Verification items for the finished model (mm, model axes). A direction names the side the tool comes from. Give positions to 0.01 mm unless a question says otherwise; leave off trailing zeros. Loops run counter-clockwise (first coordinate to the right, second up) from the corner with the lowest first, then second, coordinate; pieces in that order, holes last. Notation, with made-up numbers: (74, 78.25) - (83, 78.25) arc R19 cw to (83, 95.25) - close; hole circle Ø9 at (-2.75, -27). An arc over 180 degrees is marked (long way). One line per item, written item: value. Start each with the question number.
1. Scan lines: L1, parallel to X at y = -0.1, z = 4; L2, parallel to Z at x = 14, y = -0.7; L3, parallel to Z at x = 13, y = 0. Record each from-to range of solid material in increasing order. Write a range as [from, to].
2. Sectioned sample at A-A (x = 14). Record the cut outline in (y, z), plus the area to 3 significant figures.
3. Sectioned sample at D-D (x = 7). Record the cut outline in (y, z).
4. Access from +Z, -Z, +X, -X, +Y, -Y to the whole of each face (thin tool, end or side, straight path). Record for faces 4 (the cylindrical face through (-2.44, 7.94, -0.54)), 5 (the flat face through (16.5, 0, 0)).
5. Sectioned sample at B-B (z = -5.5). Record the cut outline in (x, y), plus the area to 3 significant figures.
6. Mould release check, pull along Z, two halves, no side actions. Record for faces 1 (the flat face through (0, 12, 0)), 2 (the cylindrical face through (-12.648, 0.028, -5.474)), 3 (the flat face through (0, 0, 10)): pulls with the +Z half, pulls with the -Z half, needs draft (parallel to the pull), parting line crosses it, or undercut.
7. Sectioned sample at C-C (y = 5.25). Record the cut outline in (x, z), plus the area to 3 significant figures.
8. Gauge pin test, flat end, axial feed: pin 1 (10 mm diameter, centred on x = 7.5, z = -6, fed in from +Y). Record the tip position at first contact, or that the pin passes through.
from build123d import *

# Parameters (mm, degrees)
SKETCH1_W           = 33
SKETCH1_H           = 20
BOSS_EXTRUDE1_DEPTH = 2
SKETCH2_R           = 2
CUT_EXTRUDE1_DEPTH  = 20.704060495
SKETCH3_R           = 2.5
BOSS_EXTRUDE2_DEPTH = 10
FILLET1_SIZE        = 2


with BuildPart() as part:
    # Sketch1 → Boss-Extrude1 (new, symmetric)
    with BuildSketch(Plane(origin=(0, 0, 0), x_dir=(1, 0, 0), z_dir=(0, 1, 0))):
        Rectangle(SKETCH1_W, SKETCH1_H)
    extrude(amount=BOSS_EXTRUDE1_DEPTH, both=True)

    # Sketch2 → Cut-Extrude1 (cut, through all)
    with BuildSketch(Plane(origin=(0, 2, 0), x_dir=(1, 0, 0), z_dir=(0, 1, 0))):
        with Locations(Location((-14, 4, 0), (0, 0, 270))):
            Circle(SKETCH2_R)
        with Locations(Location((-14, -4, 0), (0, 0, 270))):
            Circle(SKETCH2_R)
        with Locations(Location((14, -4, 0), (0, 0, 90))):
            Circle(SKETCH2_R)
        with Locations(Location((14, 4, 0), (0, 0, 90))):
            Circle(SKETCH2_R)
    extrude(amount=-CUT_EXTRUDE1_DEPTH, mode=Mode.SUBTRACT)

    # Sketch3 → Boss-Extrude2 (add)
    with BuildSketch(Plane(origin=(0, 2, 0), x_dir=(1, 0, 0), z_dir=(0, 1, 0))):
        with Locations(Location((0, 0, 0), (0, 0, 270))):
            Circle(SKETCH3_R)
    extrude(amount=BOSS_EXTRUDE2_DEPTH)

    # Fillet1
    # a fillet whose section is not a circle: 2 mm, written as the material it adds along each edge
    with BuildSketch(Plane(origin=(0, 2, 0), x_dir=(0, 0, 1), z_dir=(-1, 0, 0))) as fillet1_piece_1:
        with BuildLine():
            Bezier((2.5 + FILLET1_SIZE, 0), (2.5, 0), (2.5, FILLET1_SIZE), weights=[1, 0.141421356, 1])
            Line((2.5, FILLET1_SIZE), (2.5, 0))
            Line((2.5, 0), (2.5 + FILLET1_SIZE, 0))
        make_face()
    revolve(axis=Axis((0, 2, 0), (0, 1, 0)))


solid = part.part
Results are:
1. L1: x = [-16.5, -16], [-12, 12], [16, 16.5]
1. L2: z = [-10, -6], [-2, 2], [6, 10]
1. L3: z = [-10, -5.73], [-2.27, 2.27], [5.73, 10]
2. outline: (-2, -10) - (2, -10) - (2, -6) - (-2, -6) - close; (-2, -2) - (2, -2) - (2, 2) - (-2, 2) - close; (-2, 6) - (2, 6) - (2, 10) - (-2, 10) - close
2. area: 48.0 mm^2
3. outline: (-2, -10) - (2, -10) - (2, 10) - (-2, 10) - close
4. face 4: +Y
4. face 5: +Z, -Z, +X, +Y, -Y
5. outline: (-16.5, -2) - (-15.32, -2) - (-15.32, 2) - (-16.5, 2) - close; (-12.68, -2) - (12.68, -2) - (12.68, 2) - (-12.68, 2) - close; (15.32, -2) - (16.5, -2) - (16.5, 2) - (15.32, 2) - close
5. area: 111 mm^2
6. face 1: needs draft
6. face 2: undercut
6. face 3: pulls with the +Z half
7. outline: circle Ø5 at (0, 0)
7. area: 19.6 mm^2
8. pin 1: stops at y = 2
